Geometry check sheet. Reference: drawing and pictorial views, mm from the part's lowest x, y, z. A direction names the side the tool comes from. Round coordinates to 2 decimals unless told otherwise and drop trailing zeros. Write each loop counter-clockwise with the first axis right and the second up, starting at its lowest first coordinate (ties: lowest second). Pieces come first, ordered by that corner, then holes. Notation, with made-up numbers: (69, 19.5) - (106, 19.5) arc R23 cw to (106, 57.5) - close; hole circle Ø5 at (56.25, 59.25). An arc over 180 degrees is marked (long way). Return JSON: item names as keys, results as strings.
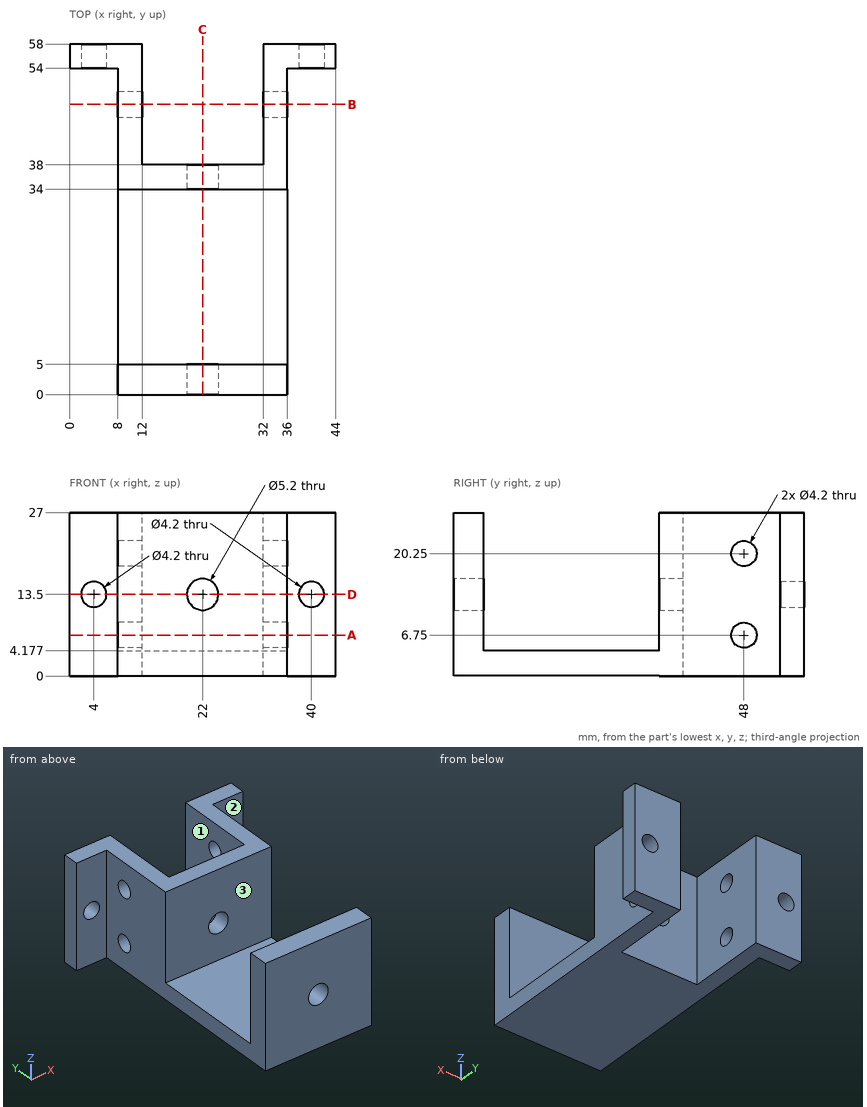
(1) Gauge pin test, flat ends, axial feed: pin 1 (22.5 mm diameter, centred on x = 25, y = 22, fed in from +Z); pin 2 (5.5 mm diameter, centred on y = 48, z = 20.25, fed in from +X); pin 3 (7 mm diameter, centred on x = 15.5, z = 17.5, fed in from -Y); pin 4 (13.5 mm diameter, centred on y = 31, z = 13.5, fed in from -X). Record the tip position at first contact, or that the pin passes through.
Response values:
{"pin 1": "stops at z = 4.18", "pin 2": "stops at x = 36", "pin 3": "stops at y = 0", "pin 4": "stops at x = 8"}
(2) Section check B-B, the plane y = 48. Enter the section's corners in (x, z), plus the area to 3 significant figures.
Response values:
{"outline": "(8, 0) - (12, 0) - (12, 4.65) - (8, 4.65) - close; (8, 8.85) - (12, 8.85) - (12, 18.15) - (8, 18.15) - close; (8, 22.35) - (12, 22.35) - (12, 27) - (8, 27) - close; (32, 0) - (36, 0) - (36, 4.65) - (32, 4.65) - close; (32, 8.85) - (36, 8.85) - (36, 18.15) - (32, 18.15) - close; (32, 22.35) - (36, 22.35) - (36, 27) - (32, 27) - close", "area": "149 mm^2"}
(3) Access from +Z, -Z, +X, -X, +Y, -Y to the whole of each face (thin tool, end or side, straight path). Record for the marked faces 1, 2 and 3.
Response values:
{"face 1": "+Z, -Z, +Y", "face 2": "+Z, -Z, +X, -Y", "face 3": "+Z, +X, -X"}
(4) Section check C-C, the plane x = 22. Enter the section's corners in (y, z), plus the area to 3 significant figures.
Response values:
{"outline": "(0, 0) - (38, 0) - (38, 10.9) - (34, 10.9) - (34, 4.18) - (5, 4.18) - (5, 10.9) - (0, 10.9) - close; (0, 16.1) - (5, 16.1) - (5, 27) - (0, 27) - close; (34, 16.1) - (38, 16.1) - (38, 27) - (34, 27) - close", "area": "317 mm^2"}
(5) Section check D-D, the plane z = 13.5. Give the number of separate pieces and of enclosed holes in the cut face.
Response values:
{"separate pieces": "6", "enclosed holes": "0"}
(6) Section check A-A, the plane z = 6.75. Enter the section's corners in (x, y).
Response values:
{"outline": "(0, 54) - (8, 54) - (8, 50.1) - (12, 50.1) - (12, 58) - (0, 58) - close; (8, 0) - (36, 0) - (36, 5) - (8, 5) - close; (8, 34) - (36, 34) - (36, 45.9) - (32, 45.9) - (32, 38) - (12, 38) - (12, 45.9) - (8, 45.9) - close; (32, 50.1) - (36, 50.1) - (36, 54) - (44, 54) - (44, 58) - (32, 58) - close"}
(7) Material ranges on line 1 along Z through (x, y) = (33, 48); line 2 along X through (y, z) = (52, 8.5); line 3 along Y through (x, z) = (22, 9), recorded low to high. Write a range as [from, to].
Response values:
{"line 1": "z = [0, 4.65], [8.85, 18.15], [22.35, 27]", "line 2": "x = [8, 12], [32, 36]", "line 3": "y = [0, 5], [34, 38]"}
